Here's how the part is built. I have some questions about the finished solid (model axes, mm). A direction names the side the tool comes from. Give positions to 0.01 mm unless a question says otherwise; leave off trailing zeros. Write each loop counter-clockwise with the first axis right and the second up, starting at its lowest first coordinate (ties: lowest second). Pieces come first, ordered by that corner, then holes. Notation, with made-up numbers: M -9.75,-7 L 36.25,-7 A26 ccw 36.25,26 Z; hole C 21,14 d6. An arc over 180 degrees is marked long. Use one line per item in the form item = value. Start each with the question number.
Autodesk Inventor part; units mm, degrees
ref_plane "YZ Plane" through (0, 0, 0) normal (1, 0, 0) x (0, 1, 0)
ref_plane "XZ Plane" through (0, 0, 0) normal (0, 1, 0) x (-1, 0, 0)
ref_plane "XY Plane" through (0, 0, 0) normal (0, 0, 1) x (1, 0, 0)
sketch "Sketch1" plane through (0, 0, 0) normal (0, 1, 0) x (-1, 0, 0)
  line L0 (0, 0) -> (5.5, 0)
  line L1 (5.5, 0) -> (5.5, -5.5)
  line L2 (5.5, -5.5) -> (0, -5.5)
  line L3 (0, -5.5) -> (0, 0)
  dimension "d0" = 5.5
  dimension "d1" = 5.5
extrude "Extrusion1" add sketch "Sketch1" along normal blind 9.5
sketch "Sketch2" plane through (0, 9.5, 0) normal (0, 1, 0) x (1, 0, 0)
  line L0 (-5.5, 5.5) -> (-5.5, 0)
  line L1 (-5.5, 2.75) -> (0, 2.75)
  line L2 (-2.75, 5.5) -> (-2.75, 0)
  line L3 (7.5, -7.5) -> (-13, -7.5)
  line L4 (-13, -7.5) -> (-13, 13)
  line L5 (-13, 13) -> (7.5, 13)
  line L6 (7.5, 13) -> (7.5, -7.5)
  line L7 (7.5, -7.5) -> (-13, 13) construction
  line L8 (-13, -7.5) -> (7.5, 13) construction
  point P0 (0, 0)
  point P1 (-2.75, 2.75)
  dimension "d4" = 20.5
  dimension "d5" = 20.5
extrude "Extrusion2" add sketch "Sketch2" along normal blind 2
sketch "Sketch4" plane through (7.5, 9.5, 7.5) normal (1, 0, 0) x (0, 0, -1)
  line L0 (0, 2) -> (20.5, 2)
  line L1 (20.5, 2) -> (20.5, 5)
  circle A0 centre (20.5, 5) radius 4
  point P0 (7.5, -9.5)
  dimension "d8" = 3
extrude "Extrusion3" add sketch "Sketch4" against normal blind 20.5
hole "Hole1" at (-13, 14.5, -13) direction (1, 0, 0) diameter 3 end through all
sketch "Sketch5" plane through (-13, 9.5, 7.5) normal (0, 0, 1) x (1, 0, 0)
  line L0 (0, 2) -> (20.5, 2)
  line L1 (6.5, 2) -> (14, 2)
  line L2 (14, 2) -> (14, 14.1899)
  line L3 (14, 14.1899) -> (6.5, 14.1899)
  line L4 (6.5, 14.1899) -> (6.5, 2)
  line L5 (0, 9) -> (0, 1)
  line L6 (20.5, 9) -> (20.5, 1)
  point P0 (13, -9.5)
  dimension "d20" = 12.1899
  dimension "d21" = 6.5
  dimension "d22" = 6.5
  dimension "d23" = 7.5
extrude "Extrusion4" cut sketch "Sketch5" against normal blind 30
properties part number "camera holder"
1) On a 3-axis mill with a long thin cutter (end or side, diameter ignored), from which of +Z, -Z, +X, -X, +Y, -Y can I reach the whole of each face in a straight line? I mean faces 1 (the face through (-6.5, 16, -14)), 2 (the face through (-3, 10, -13)), 3 (the face through (0, 5, -3)), 4 (the face through (-3, 10, 7.5)), 5 (the face through (-5.5, 5, -3)). Say none if no direction works.
2) Suppose I cut it at C-C, the plane z = -1.25. List the corners of the cut face in (x, y) for me.
3) Suppose I cut it at A-A, the plane y = 14.5. List the corners of the cut face in (x, z) for me.
4) Suppose I cut it at B-B, the plane x = -3.5. List the corners of the cut face in (y, z) for me, and give its area (3 significant figures).
5) Thinking about a two-plate mould opening in Z: for faces 6 (the face through (-3, 5, -5.5)), 7 (the face through (4.3, 14.43, -14.5)), 8 (the face through (-3, 5, 0)), which applies, released by +Z, released by -Z, zero draft, split by the parting line, or undercut?
6) Please list where these lines run through material, in increasing order: line 1 (Z direction, x = -9.5, y = 14.5); line 2 (X direction, y = 13.5, z = -14.75); line 3 (X direction, y = 6.75, z = -0.25).
7) Suppose I cut it at D-D, the plane x = -9. List the corners of the cut face in (y, z) for me.
8) Will these pins go through, and if not, where does the flat tip stop? P1, Ø4.5, axis at y = 3, z = -3.5, coming from the -X side; P2, Ø6, axis at x = 0.5, z = -7, coming from the +Y side; P3, Ø1, axis at x = -1, z = -5, coming from the -Y side; P4, Ø6, axis at x = -2, y = 4, coming from the -Z side.
Checks:
q1.face_1 = +Z, -Z, +Y
q1.face_2 = -Z, +X, -X, -Y
q1.face_3 = +Z, -Z, +X, -Y
q1.face_4 = +Z, +X, -X, +Y, -Y
q1.face_5 = +Z, -Z, -X, -Y
q2.outline = M -13,9.5 L -5.5,9.5 L -5.5,0 L 0,0 L 0,9.5 L 7.5,9.5 L 7.5,11.5 L -13,11.5 Z
q3.outline = M -13,-17 L -6.5,-17 L -6.5,-14.5 L -13,-14.5 Z; M -13,-11.5 L -6.5,-11.5 L -6.5,-9 L -13,-9 Z; M 1,-17 L 7.5,-17 L 7.5,-14.5 L 1,-14.5 Z; M 1,-11.5 L 7.5,-11.5 L 7.5,-9 L 1,-9 Z
q4.outline = M 0,-5.5 L 9.5,-5.5 L 9.5,-13 L 10.5,-13 A4 ccw 11.5,-15.65 L 11.5,7.5 L 9.5,7.5 L 9.5,0 L 0,0 Z
q4.area = 95.1 mm^2
q5.face_6 = released by -Z
q5.face_7 = undercut
q5.face_8 = released by +Z
q6.line_1 = -17 to -14.5, -11.5 to -9
q6.line_2 = -13 to -6.5, 1 to 7.5
q6.line_3 = -5.5 to 0
q7.outline = M 9.5,-13 L 10.5,-13 A4 ccw long 11.5,-10.35 L 11.5,7.5 L 9.5,7.5 Z; hole C 14.5,-13 d3
q8.P1 = -5.5
q8.P2 = 17.1
q8.P3 = 0
q8.P4 = -5.5
